Build history of the part. All positions in model axes, mm. Face numbers are marked on the shaded views. A direction names the side the tool comes from. Give positions to 0.01 mm unless a question says otherwise; leave off trailing zeros. Order: outer loops, then holes, each group sorted by start corner. A loop starts at its lowest first (then second) coordinate and runs counter-clockwise, first axis right, second up. Notation, with made-up numbers: M 86,46 L 141,46 A10 cw 141,56 Z; hole C 70,-12 d6. An arc over 180 degrees is marked long. Answer as CSV lines item,"result".
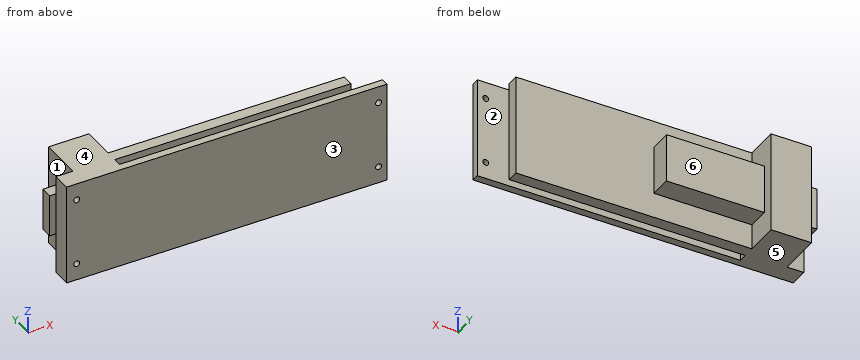
from build123d import *

# Parameters (mm, degrees)
SKETCH1_W           = 190
SKETCH1_H           = 60
SKETCH1_R           = 1.75
BOSS_EXTRUDE1_DEPTH = 4.5
SKETCH2_W           = 10
SKETCH2_H           = 60
BOSS_EXTRUDE2_DEPTH = 6.5
SKETCH3_W           = 24
SKETCH3_H           = 60
BOSS_EXTRUDE3_DEPTH = 32
SKETCH5_W           = 20
SKETCH5_H           = 25
BOSS_EXTRUDE4_DEPTH = 7
SKETCH6_W           = 140
SKETCH6_H           = 60
BOSS_EXTRUDE5_DEPTH = 7
SKETCH7_W           = 58
SKETCH7_H           = 28.953821303
BOSS_EXTRUDE6_DEPTH = 13
SKETCH8_R           = 1.75
CUT_EXTRUDE1_DEPTH  = 13


with BuildPart() as part:
    # Sketch1 → Boss-Extrude1 (new body)
    with BuildSketch(Plane(origin=(0, 0, 0), x_dir=(1, 0, 0), z_dir=(0, 1, 0))):
        Rectangle(SKETCH1_W, SKETCH1_H)
        with Locations(Location((90, -20, 0), (0, 0, 270))):
            Circle(SKETCH1_R, mode=Mode.SUBTRACT)
        with Locations(Location((90, 20, 0), (0, 0, 270))):
            Circle(SKETCH1_R, mode=Mode.SUBTRACT)
    extrude(amount=BOSS_EXTRUDE1_DEPTH)

    # Sketch2 → Boss-Extrude2 (add)
    with BuildSketch(Plane(origin=(0, 4.5, 0), x_dir=(1, 0, 0), z_dir=(0, 1, 0))):
        with Locations((-90, 0)):
            Rectangle(SKETCH2_W, SKETCH2_H)
    extrude(amount=BOSS_EXTRUDE2_DEPTH)

    # Sketch3 → Boss-Extrude3 (add)
    with BuildSketch(Plane(origin=(0, 4.5, 0), x_dir=(1, 0, 0), z_dir=(0, 1, 0))):
        with Locations((-73, 0)):
            Rectangle(SKETCH3_W, SKETCH3_H)
    extrude(amount=BOSS_EXTRUDE3_DEPTH)

    # Sketch5 → Boss-Extrude4 (add)
    with BuildSketch(Plane(origin=(0, 19, 0), x_dir=(1, 0, 0), z_dir=(0, 1, 0))):
        with Locations((-84.226759087, -0.419143158)):
            Rectangle(SKETCH5_W, SKETCH5_H)
    extrude(amount=BOSS_EXTRUDE4_DEPTH)

    # Sketch6 → Boss-Extrude5 (add)
    with BuildSketch(Plane(origin=(0, 9.5, 0), x_dir=(1, 0, 0), z_dir=(0, 1, 0))):
        with Locations((9, 0)):
            Rectangle(SKETCH6_W, SKETCH6_H)
    extrude(amount=BOSS_EXTRUDE5_DEPTH)

    # Sketch7 → Boss-Extrude6 (add)
    with BuildSketch(Plane(origin=(0, 16.5, 0), x_dir=(1, 0, 0), z_dir=(0, 1, 0))):
        with Locations((-32, 0.523089349)):
            Rectangle(SKETCH7_W, SKETCH7_H)
    extrude(amount=BOSS_EXTRUDE6_DEPTH)

    # Sketch8 → Cut-Extrude1 (cut)
    with BuildSketch(Plane.XZ):
        with Locations(Location((-89, -20, 0), (0, 0, 270))):
            Circle(SKETCH8_R)
        with Locations(Location((-89, 19.955464874, 0), (0, 0, 270))):
            Circle(SKETCH8_R)
    extrude(amount=-CUT_EXTRUDE1_DEPTH, mode=Mode.SUBTRACT)


solid = part.part
Item 1: Band-saw the part on A-A (x = -11). Give the cut face in (y, z).
Geometry says:
outline,"M 0,-30 L 4.5,-30 L 4.5,30 L 0,30 Z; M 9.5,-30 L 16.5,-30 L 16.5,-15 L 29.5,-15 L 29.5,13.95 L 16.5,13.95 L 16.5,30 L 9.5,30 Z"
Item 2: Pull direction Y, two halves, no side cores. Call the marked faces 1, 2, 3 and 4: released by +Y, released by -Y, zero draft, split by the parting line, or undercut.
Geometry says:
face 1,"undercut"
face 2,"undercut"
face 3,"released by -Y"
face 4,"zero draft"
Item 3: Drop flat-ended pins along their axis: pin 1 (6 mm diameter, centred on y = 14.5, z = 9, fed in from -X); pin 2 (4.5 mm diameter, centred on x = -89, z = 19.96, fed in from +Y); pin 3 (20.5 mm diameter, centred on y = 25.5, z = -11, fed in from -X); pin 4 (2 mm diameter, centred on x = -89, z = -20, fed in from +Y). Give the stop position or say it passes through.
Geometry says:
pin 1,"stops at x = -85"
pin 2,"stops at y = 11"
pin 3,"stops at x = -94.23"
pin 4,"passes through"
Item 4: Probe line 1 along Z through (x, y) = (90, 1.7); line 2 along X through (y, z) = (2.9, 20); line 3 along Y through (x, z) = (44.5, 5.5). List the from-to ranges inside material, lowest first. Write a range as from..to.
Geometry says:
line 1,"z = -30..-21.75, -18.25..18.25, 21.75..30"
line 2,"x = -95..-90.75, -87.25..88.25, 91.75..95"
line 3,"y = 0..4.5, 9.5..16.5"
Item 5: 3-axis set-ups, long thin cutter, end or side, ignore diameter. For the marked faces 5 and 6: which of +Z, -Z, +X, -X, +Y, -Y reach the whole face in a straight line?
Geometry says:
face 5,"-Z, +X, -X, +Y, -Y"
face 6,"+Z, -Z, +X, +Y"
Item 6: Band-saw the part on B-B (x = -89). Give the cut face in (y, z), and give its area (3 significant figures).
Geometry says:
outline,"M 0,-30 L 11,-30 L 11,-21.75 L 0,-21.75 Z; M 0,-18.25 L 11,-18.25 L 11,18.21 L 0,18.21 Z; M 0,21.71 L 11,21.71 L 11,30 L 0,30 Z; M 19,-12.08 L 26,-12.08 L 26,12.92 L 19,12.92 Z"
area,"758 mm2"
Item 7: Band-saw the part on D-D (z = 20). Give the cut face in (x, y), and give its area (3 significant figures).
Geometry says:
outline,"M -95,0 L -90.75,0 L -90.75,11 L -95,11 Z; M -87.25,0 L 88.25,0 L 88.25,4.5 L -61,4.5 L -61,9.5 L 79,9.5 L 79,16.5 L -61,16.5 L -61,36.5 L -85,36.5 L -85,11 L -87.25,11 Z; M 91.75,0 L 95,0 L 95,4.5 L 91.75,4.5 Z"
area,"2,610 mm2"
Item 8: Band-saw the part on C-C (z = -7). Give the cut face in (x, y), and give its area (3 significant figures).
Geometry says:
outline,"M -95,0 L 95,0 L 95,4.5 L -61,4.5 L -61,9.5 L 79,9.5 L 79,16.5 L -3,16.5 L -3,29.5 L -61,29.5 L -61,36.5 L -85,36.5 L -85,26 L -94.23,26 L -94.23,19 L -85,19 L -85,11 L -95,11 Z"
area,"3,490 mm2"
